```python
from build123d import *

# Parameters (mm, degrees)
OG_BASE_DEPTH       = 3
SKETCH5_R           = 1.15
CUT_EXTRUDE1_DEPTH  = 3
SKETCH6_W           = 50
SKETCH6_H           = 25
BOSS_EXTRUDE3_DEPTH = 75
SKETCH8_W           = 17
SKETCH8_H           = 58
BOSS_EXTRUDE4_DEPTH = 50
SKETCH10_W          = 45
SKETCH10_H          = 10
BOSS_EXTRUDE5_DEPTH = 35.5
SKETCH11_W          = 40.26
SKETCH11_H          = 1.8
CUT_EXTRUDE2_DEPTH  = 40
SKETCH13_W          = 38
SKETCH13_H          = 4.1
CUT_EXTRUDE3_DEPTH  = 40
SKETCH14_W          = 31.5
SKETCH14_H          = 4.1
CUT_EXTRUDE4_DEPTH  = 40
SKETCH19_R          = 7.65
CUT_EXTRUDE6_DEPTH  = 28
SKETCH21_W          = 41.177647426
SKETCH21_H          = 18.949912373
CUT_EXTRUDE7_DEPTH  = 17


with BuildPart() as part:
    # Sketch3 → OG base (new body)
    with BuildSketch(Plane(origin=(0, 0, 0), x_dir=(1, 0, 0), z_dir=(0, 1, 0))):
        Polygon((-41.21875, 24.460069444), (38.78125, 24.460069444), (38.78125, 7.460069444), (23.78125, 7.460069444), (23.78125, -0.539930556), (-26.21875, -0.539930556), (-26.21875, 7.460069444), (-41.21875, 7.460069444), align=None)
    extrude(amount=OG_BASE_DEPTH)

    # Sketch5 → Cut-Extrude1 (cut)
    with BuildSketch(Plane(origin=(0, 3, 0), x_dir=(1, 0, 0), z_dir=(0, 1, 0))):
        with Locations(Location((-37.71875, 14.760831394, 0), (0, 0, 270))):
            Circle(SKETCH5_R)
        with Locations(Location((35.28125, 14.760831394, 0), (0, 0, 270))):
            Circle(SKETCH5_R)
    extrude(amount=-CUT_EXTRUDE1_DEPTH, mode=Mode.SUBTRACT)

    # Sketch6 → Boss-Extrude3 (add)
    with BuildSketch(Plane(origin=(0, 3, 0), x_dir=(1, 0, 0), z_dir=(0, 1, 0))):
        with Locations((-1.21875, 11.960069444)):
            Rectangle(SKETCH6_W, SKETCH6_H)
    extrude(amount=BOSS_EXTRUDE3_DEPTH)

    # Sketch8 → Boss-Extrude4 (add)
    with BuildSketch(Plane.ZY.offset(26.21875)):
        with Locations((9.039930556, 49)):
            Rectangle(SKETCH8_W, SKETCH8_H)
    extrude(amount=-BOSS_EXTRUDE4_DEPTH)

    # Sketch10 → Boss-Extrude5 (add)
    with BuildSketch(Plane(origin=(0, 0, -24.460069444), x_dir=(-1, 0, 0), z_dir=(0, 0, -1))):
        with Locations((1.21875, 58.965562055)):
            Rectangle(SKETCH10_W, SKETCH10_H)
    extrude(amount=BOSS_EXTRUDE5_DEPTH)

    # Sketch11 → Cut-Extrude2 (cut)
    with BuildSketch(Plane(origin=(0, 0, -59.960069444), x_dir=(-1, 0, 0), z_dir=(0, 0, -1))):
        with Locations((1.21875, 58.965562055)):
            Rectangle(SKETCH11_W, SKETCH11_H)
    extrude(amount=-CUT_EXTRUDE2_DEPTH, mode=Mode.SUBTRACT)

    # Sketch13 → Cut-Extrude3 (cut)
    with BuildSketch(Plane(origin=(0, 0, -59.960069444), x_dir=(-1, 0, 0), z_dir=(0, 0, -1))):
        with Locations((1.21875, 56.015562055)):
            Rectangle(SKETCH13_W, SKETCH13_H)
    extrude(amount=-CUT_EXTRUDE3_DEPTH, mode=Mode.SUBTRACT)

    # Sketch14 → Cut-Extrude4 (cut)
    with BuildSketch(Plane(origin=(0, 0, -59.960069444), x_dir=(-1, 0, 0), z_dir=(0, 0, -1))):
        with Locations((-0.03125, 61.915562055)):
            Rectangle(SKETCH14_W, SKETCH14_H)
    extrude(amount=-CUT_EXTRUDE4_DEPTH, mode=Mode.SUBTRACT)

    # Sketch19 → Cut-Extrude6 (cut)
    with BuildSketch(Plane(origin=(0, 78, 0), x_dir=(1, 0, 0), z_dir=(0, 1, 0))):
        with Locations(Location((0, 10.366835576, 0), (0, 0, 270))):
            Circle(SKETCH19_R)
    extrude(amount=-CUT_EXTRUDE6_DEPTH, mode=Mode.SUBTRACT)

    # Sketch21 → Cut-Extrude7 (cut)
    with BuildSketch(Plane.XY.offset(17.539930556)):
        with Locations((-1.21875, 35.722177319)):
            Rectangle(SKETCH21_W, SKETCH21_H)
    extrude(amount=-CUT_EXTRUDE7_DEPTH, mode=Mode.SUBTRACT)


solid = part.part
```
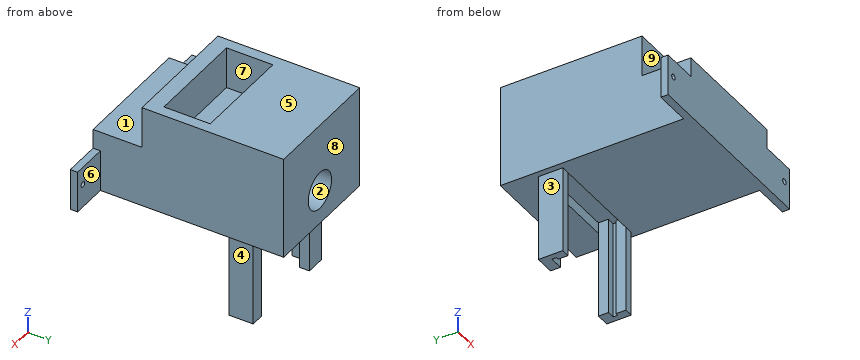
Work out the finished part from the listing and answer in its coordinate system (mm). Face numbers are marked on the shaded views. A direction names the side the tool comes from. Coordinates: 2 decimals unless noted, no trailing zeros. Loops run counter-clockwise (first coordinate to the right, second up) from the corner with the lowest first, then second, coordinate; pieces in that order, holes last. Notation, with made-up numbers: (-39.75, -31.5) - (-27.75, -31.5) arc R26 cw to (-27.75, -6.5) - close; hole circle Ø9 at (79.25, 16). An arc over 180 degrees is marked (long way). Use a Markdown table: item, result.
Item 1: Find section C-C, the plane z = -21.5. Determine the outline of the cut face in (x, y).
Evaluation:
| item | result |
|---|---|
| outline | (-41.22, 0) - (38.78, 0) - (38.78, 3) - (23.78, 3) - (23.78, 78) - (-26.22, 78) - (-26.22, 3) - (-41.22, 3) - close; hole (-21.35, 58.07) - (-20.22, 58.07) - (-20.22, 53.97) - (17.78, 53.97) - (17.78, 58.07) - (18.91, 58.07) - (18.91, 59.87) - (15.78, 59.87) - (15.78, 63.97) - (-15.72, 63.97) - (-15.72, 59.87) - (-21.35, 59.87) - close |
Item 2: The mould has two halves that part along X. Classify the marked faces 1, 2, 3 and 4: +X half, -X half, draft (parallel to the pull), parting line (faces both ways), or undercut.
Evaluation:
| item | result |
|---|---|
| face 1 | draft |
| face 2 | undercut |
| face 3 | -X half |
| face 4 | +X half |
Item 3: Given pin 1 Ø4.5 at (x, z) = (1, -14) entering from +Y; pin 2 Ø1.2 at (x, z) = (-21, -40) entering from +Y; pin 3 Ø4.5 at (y, z) = (56, -42.5) entering from -X, each flat-ended and moving along its own axis, determine where each tip first touches the part or whether it passes through.
Evaluation:
| item | result |
|---|---|
| pin 1 | stops at y = 50 |
| pin 2 | stops at y = 63.97 |
| pin 3 | stops at x = -23.72 |
Item 4: Consider probe 1 along Y at (x, z) = (-20.5, -49.5); probe 2 along Y at (x, z) = (-5.5, -23); probe 3 along X at (y, z) = (58.5, -32). Determine where each line is inside the solid, lowest interval first. Write a range as from..to.
Evaluation:
| item | result |
|---|---|
| probe 1 | y = 53.97..58.07, 59.87..63.97 |
| probe 2 | y = 0..53.97, 63.97..78 |
| probe 3 | x = -23.72..-21.35, 18.91..21.28 |
Item 5: Find section D-D, the plane y = 43. Determine the outline of the cut face in (x, z).
Evaluation:
| item | result |
|---|---|
| outline | (-26.22, -24.46) - (23.78, -24.46) - (23.78, 17.54) - (19.37, 17.54) - (19.37, 0.54) - (-21.81, 0.54) - (-21.81, 17.54) - (-26.22, 17.54) - close |
Item 6: Find section A-A, the plane z = -36.5. Determine the outline of the cut face in (x, y), and give its area (3 significant figures).
Evaluation:
| item | result |
|---|---|
| outline | (-23.72, 53.97) - (-20.22, 53.97) - (-20.22, 58.07) - (-21.35, 58.07) - (-21.35, 59.87) - (-15.72, 59.87) - (-15.72, 63.97) - (-23.72, 63.97) - close; (15.78, 59.87) - (18.91, 59.87) - (18.91, 58.07) - (17.78, 58.07) - (17.78, 53.97) - (21.28, 53.97) - (21.28, 63.97) - (15.78, 63.97) - close |
| area | 92.6 mm2 |
Item 7: For the marked faces 5, 6, 7, 8 and 9, determine the directions among +Z, -Z, +X, -X, +Y, -Y from which every point of the face is accessible in a straight line to the end or side of a thin tool.
Evaluation:
| item | result |
|---|---|
| face 5 | +Z, +X, -X, +Y, -Y |
| face 6 | +Z, -Z, +X, +Y |
| face 7 | +Z |
| face 8 | +Z, -Z, +X, -X, +Y |
| face 9 | +Z, +X, -X, -Y |
Item 8: Find section B-B, the plane x = 12. Determine the outline of the cut face in (y, z).
Evaluation:
| item | result |
|---|---|
| outline | (0, -24.46) - (53.97, -24.46) - (53.97, -19.96) - (63.97, -19.96) - (63.97, -24.46) - (78, -24.46) - (78, 17.54) - (45.2, 17.54) - (45.2, 0.54) - (26.25, 0.54) - (26.25, 17.54) - (20, 17.54) - (20, 0.54) - (0, 0.54) - close |
